Source: three-view drawing plus pictorial views. Frame: mm from the lowest corner of the part. Coordinates: 2 decimals unless noted, no trailing zeros. Loops run counter-clockwise (first coordinate to the right, second up) from the corner with the lowest first, then second, coordinate; pieces in that order, holes last. Notation, with made-up numbers: M -13,56 L 13,56 A16 ccw 13,76 Z; hole C 35.5,84 d4. An arc over 180 degrees is marked long. Use a Markdown table: item, result. Add a question column.
1. Pin query (flat end, axial travel): pin 1 (1 mm diameter, centred on y = 9, z = 19.5, fed in from -X); pin 2 (6 mm diameter, centred on x = 4, y = 7, fed in from +Z) (1 decimal). Return the tip coordinate at first contact, or that it passes through.
2. Section B-B on y = 9.25. Output: boundary loops of the cut face in (x, z), then the cut area to 3 significant figures.
3. Draft query along X for the marked faces 1, 2 and 3. Return one class per face: +X half, -X half, draft (parallel to the pull), parting line (faces both ways), or undercut.
4. Line query: L1, parallel to X at y = 9, z = 13.75 (1 decimal); L2, parallel to X at y = 11.25, z = 7 (1 decimal); L3, parallel to Z at x = 15, y = 3.25 (1 decimal). Output: solid intervals per line, ascending. Write a range as [from, to].
5. Section C-C on y = 10.5. Output: boundary loops of the cut face in (x, z).
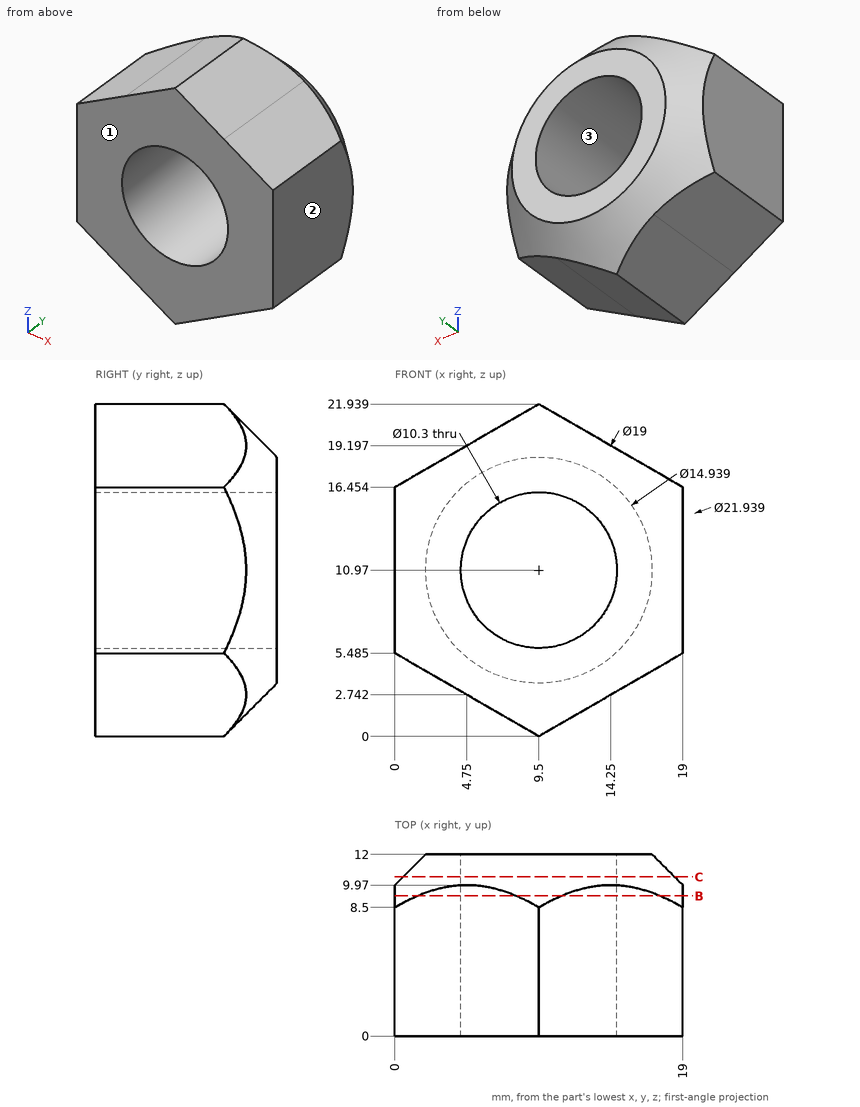
Answers below:
| question | item | result |
|---|---|---|
| 1 | pin 1 | stops at x = 4.41 |
| 1 | pin 2 | stops at z = 20.5 |
| 2 | outline | M 0,7.2 A10.22 ccw 1.49,4.63 L 8.01,0.86 A10.22 ccw 10.99,0.86 L 17.51,4.63 A10.22 ccw 19,7.2 L 19,14.74 A10.22 ccw 17.51,17.31 L 10.99,21.08 A10.22 ccw 8.01,21.08 L 1.49,17.31 A10.22 ccw 0,14.74 Z; hole C 9.5,10.97 d10.3 |
| 2 | area | 223 mm² |
| 3 | face 1 | draft |
| 3 | face 2 | +X half |
| 3 | face 3 | undercut |
| 4 | L1 | x = [0, 5.2], [13.8, 19] |
| 4 | L2 | x = [2.3, 6.2], [12.8, 16.7] |
| 4 | L3 | z = [3.2, 18.8] |
| 5 | outline | C 9.5,10.97 d17.94; hole C 9.5,10.97 d10.3 |
